Job drawing, mm, ordinate dimensions from the low corner. One solid piece. A direction names the side the tool comes from. Round coordinates to 2 decimals unless told otherwise and drop trailing zeros. Loops run counter-clockwise (first coordinate to the right, second up) from the corner with the lowest first, then second, coordinate; pieces in that order, holes last. Notation, with made-up numbers: M 42,86.5 L 57,86.5 A26 ccw 57,123.5 Z; hole C -22.75,83.5 d3. An arc over 180 degrees is marked long. Put each result on its own line as item: value. Start each with the question number.
1) Slice it at B-B on z = 71. Give the cut face in (x, y) (1 decimal).
2) Slice it at D-D on x = 5. Give the cut face in (y, z) (1 decimal), then the cut area to 3 significant figures.
3) Drop flat-ended pins along their axis: pin 1 Ø1 at (y, z) = (12.5, 22) entering from -X; pin 2 Ø4 at (x, z) = (25, 71) entering from -Y (1 decimal); pin 3 Ø8 at (x, y) = (13.5, 32) entering from -Z. Give the stop position or say it passes through.
4) Probe line 1 along X through (y, z) = (63, 44.5); line 2 along Z through (x, y) = (25, 45.5) (1 decimal); line 3 along Y through (x, z) = (31.5, 48). List the from-to ranges inside material, lowest first.
5) Slice it at C-C on y = 27.5. Give the cut face in (x, z), then the cut area to 3 significant figures.
6) Which spindle directions (+Z, -Z, +X, -X, +Y, -Y) get a long thin tool onto all of the face, cutting with end or side? Do the marked faces 1 and 2. Say none if no direction does.
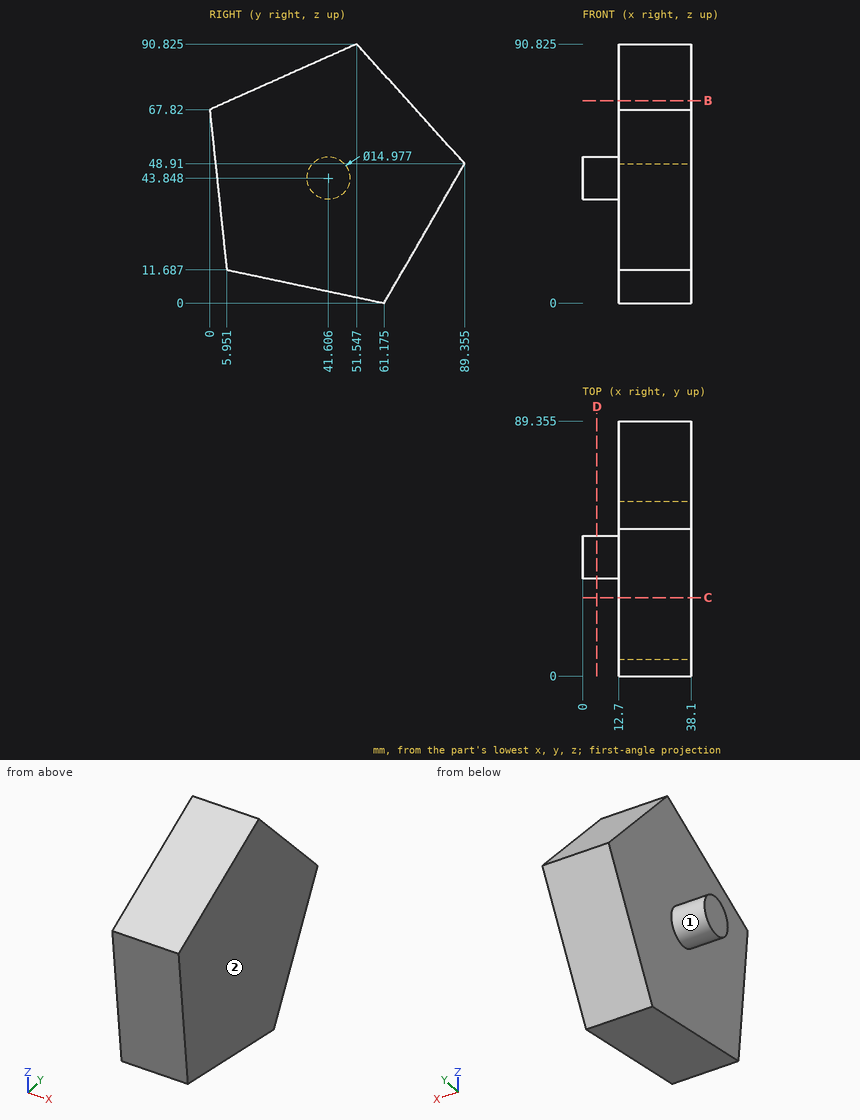
Recorded:
1. outline: M 12.7,7.1 L 38.1,7.1 L 38.1,69.4 L 12.7,69.4 Z
2. outline: C 41.6,43.8 d15
2. area: 176 mm2
3. pin 1: stops at x = 12.7
3. pin 2: stops at y = 2.6
3. pin 3: stops at z = 5.33
4. line 1: x = 12.7 to 38.1
4. line 2: z = 3.3 to 88.1
4. line 3: y = 2.1 to 88.83
5. outline: M 12.7,7.13 L 38.1,7.13 L 38.1,80.09 L 12.7,80.09 Z
5. area: 1,850 mm2
6. face 1: -X
6. face 2: +Z, -Z, +X, +Y, -Y
